Geometry: see drawing. Coordinates: mm, zero at the bounding-box minimum. A direction names the side the tool comes from. Round coordinates to 2 decimals unless told otherwise and drop trailing zeros. Order: outer loops, then holes, each group sorted by start corner. A loop starts at its lowest first (then second) coordinate and runs counter-clockwise, first axis right, second up. Notation, with made-up numbers: (42, -36.5) -> (85, -36.5) arc R15 cw to (85, -25.5) -> close; hole circle Ø10 at (17.5, 62). An arc over 180 degrees is marked (long way). Use a Markdown table: item, result.
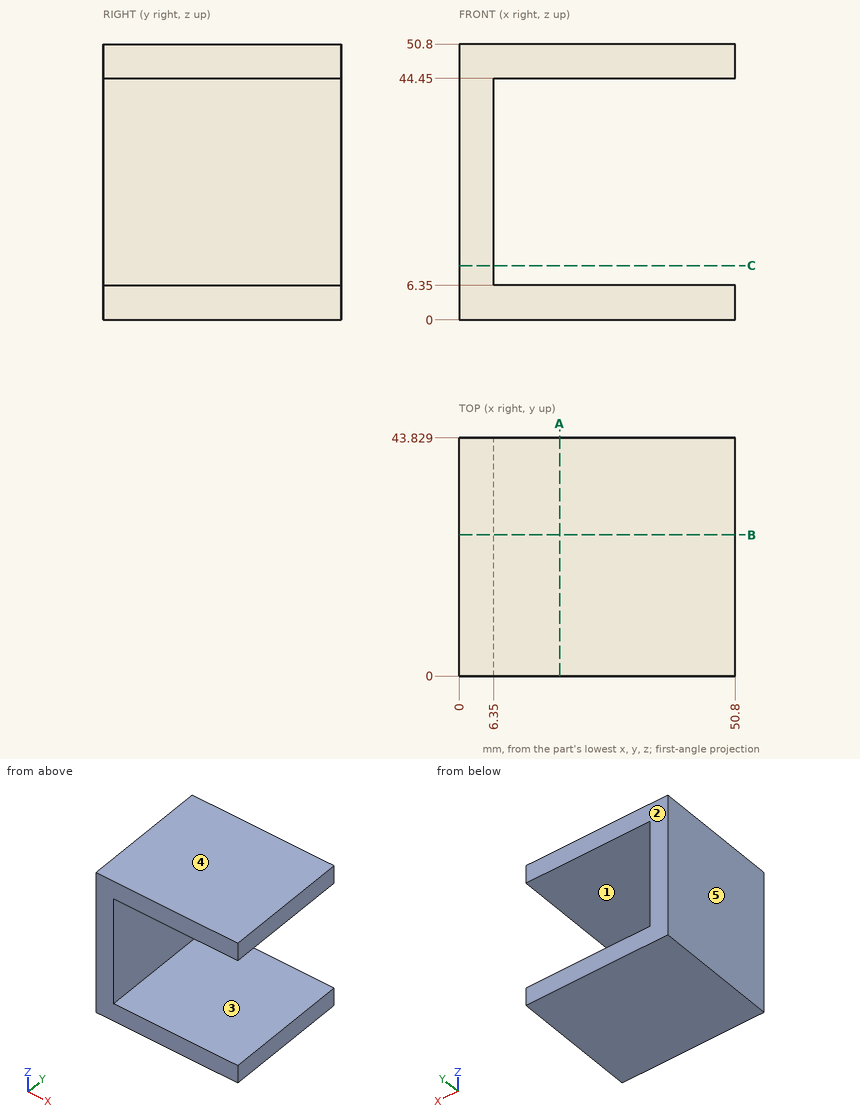
1) Cut plane B-B on y = 26. Return loops of the section in (x, z), and give its area (3 significant figures).
Answer key:
| item | result |
|---|---|
| outline | (0, 0) -> (50.8, 0) -> (50.8, 6.35) -> (6.35, 6.35) -> (6.35, 44.45) -> (50.8, 44.45) -> (50.8, 50.8) -> (0, 50.8) -> close |
| area | 887 mm^2 |
2) Set-up query: the marked faces 1 and 2. Return all of +Z, -Z, +X, -X, +Y, -Y with unobstructed straight access to the full face (end or side cutting, diameter ignored); none if empty.
Answer key:
| item | result |
|---|---|
| face 1 | +X, +Y, -Y |
| face 2 | +Z, -Z, +X, -X, +Y |
3) Cut plane C-C on z = 10. Return loops of the section in (x, y).
Answer key:
| item | result |
|---|---|
| outline | (0, 0) -> (6.35, 0) -> (6.35, 43.83) -> (0, 43.83) -> close |
4) Cut plane A-A on x = 18.5. Return loops of the section in (y, z).
Answer key:
| item | result |
|---|---|
| outline | (0, 0) -> (43.83, 0) -> (43.83, 6.35) -> (0, 6.35) -> close; (0, 44.45) -> (43.83, 44.45) -> (43.83, 50.8) -> (0, 50.8) -> close |
5) Ray query, probe 1 along Z at (x, y) = (8.5, 25); probe 2 along X at (y, z) = (10, 15). Return the intervals inside material, ascending.
Answer key:
| item | result |
|---|---|
| probe 1 | z = 0 to 6.35, 44.45 to 50.8 |
| probe 2 | x = 0 to 6.35 |
6) Draft query along Z for the marked faces 3, 4 and 5. Return one class per face: released by +Z, released by -Z, zero draft, split by the parting line, or undercut.
Answer key:
| item | result |
|---|---|
| face 3 | undercut |
| face 4 | released by +Z |
| face 5 | zero draft |
7) Contact query for a flat-ended pin moving along its axis: P1, Ø1, axis at y = 31.5, z = 41.5, coming from the +X side. Output: stop coordinate, or through.
Answer key:
| item | result |
|---|---|
| P1 | stops at x = 6.35 |
